Autodesk Inventor part; units mm, degrees
ref_plane "YZ Plane" through (0, 0, 0) normal (1, 0, 0) x (0, 1, 0)
ref_plane "XZ Plane" through (0, 0, 0) normal (0, 1, 0) x (-1, 0, 0)
ref_plane "XY Plane" through (0, 0, 0) normal (0, 0, 1) x (1, 0, 0)
sketch "Sketch1" plane through (0, 0, 0) normal (0, 0, 1) x (1, 0, 0)
  circle A0 centre (0, 0) radius 250
  circle A1 centre (0, 0) radius 210
  dimension "d0" = 500
  dimension "d1" = 420
extrude "Extrusion1" add sketch "Sketch1" along normal blind 10
sketch "Sketch2" plane through (0, 0, 10) normal (0, 0, 1) x (1, 0, 0)
  circle A0 centre (0, 0) radius 225 construction
  circle A1 centre (0, 0) radius 210
  point P0 (0, 225)
  dimension "d4" = 450
hole "Hole1" at (0, 225, 10) direction (0, 0, -1) diameter 9 end through all
pattern_circular "Circular Pattern1" count 8 over 360 about axis through (0, 0, 0) along (0, 0, 1) of "Hole1"
properties part number "Кольцо проект Алексенко"
The listing builds one solid part. Answer for the finished solid, in the listing's coordinates (mm). Coordinates: 2 decimals unless noted, no trailing zeros. Order: outer loops, then holes, each group sorted by start corner. A loop starts at its lowest first (then second) coordinate and runs counter-clockwise, first axis right, second up. Notation, with made-up numbers: M 47.25,29.5 L 101.25,29.5 A26 cw 101.25,61.5 Z; hole C 88.25,82 d1. An arc over 180 degrees is marked long. Answer as a JSON object with one key per item and string values. Group by question number.
1. Flat-ended cylindrical pins translate along their axes: P1, Ø2, axis at y = 153.5, z = 7, coming from the -X side; P2, Ø5.5, axis at x = 225, y = 0, coming from the +Z side; P3, Ø4, axis at y = -197, z = 6, coming from the +X side; P4, Ø1.5, axis at x = -177.5, z = 7.5, coming from the -Y side. Find the tip coordinate at first contact, or state that the pin passes through.
2. Section A-A on x = 193 is taken. Write down the section's boundary in (y, z).
3. Section C-C on z = 6 is taken. State how many separate pieces and enclosed holes the cut face has, then the cut area to 3 significant figures.
4. Straight lines are drawn through the part: line 1 (X direction, y = -50, z = 2); line 2 (Y direction, x = 225.5, z = 6.5); line 3 (X direction, y = 12.5, z = 2.25). For each, find the intervals that lie inside material, in ascending order.
5. Section B-B on y = -195 is taken. Write down the section's boundary in (x, z).
6. Determine the mould class of faces 1 (the flat face through (-149, 149, 10)), 2 (the cylindrical face through (-249.76, -10.99, 4.93)), 3 (the cylindrical face through (200.3, -63.08, 4.93)) for opening direction X: released by +X, released by -X, zero draft, split by the parting line, or undercut.
Values follow:
{
 "1": {"P1": "x = -198.1", "P2": "through", "P3": "x = 156.44", "P4": "y = -176.8"},
 "2": {"outline": "M -158.91,0 L -82.77,0 L -82.77,10 L -158.91,10 Z; M 82.77,0 L 158.91,0 L 158.91,10 L 82.77,10 Z"},
 "3": {"separate pieces": "1", "enclosed holes": "9", "area": "57,300 mm2"},
 "4": {"line 1": "-244.95 to -203.96, 203.96 to 244.95", "line 2": "-107.93 to -4.47, 4.47 to 107.93", "line 3": "-249.69 to -209.63, 209.63 to 249.69"},
 "5": {"outline": "M -156.44,0 L -77.94,0 L -77.94,10 L -156.44,10 Z; M 77.94,0 L 156.44,0 L 156.44,10 L 77.94,10 Z"},
 "6": {"face 1": "zero draft", "face 2": "split by the parting line", "face 3": "undercut"}
}
